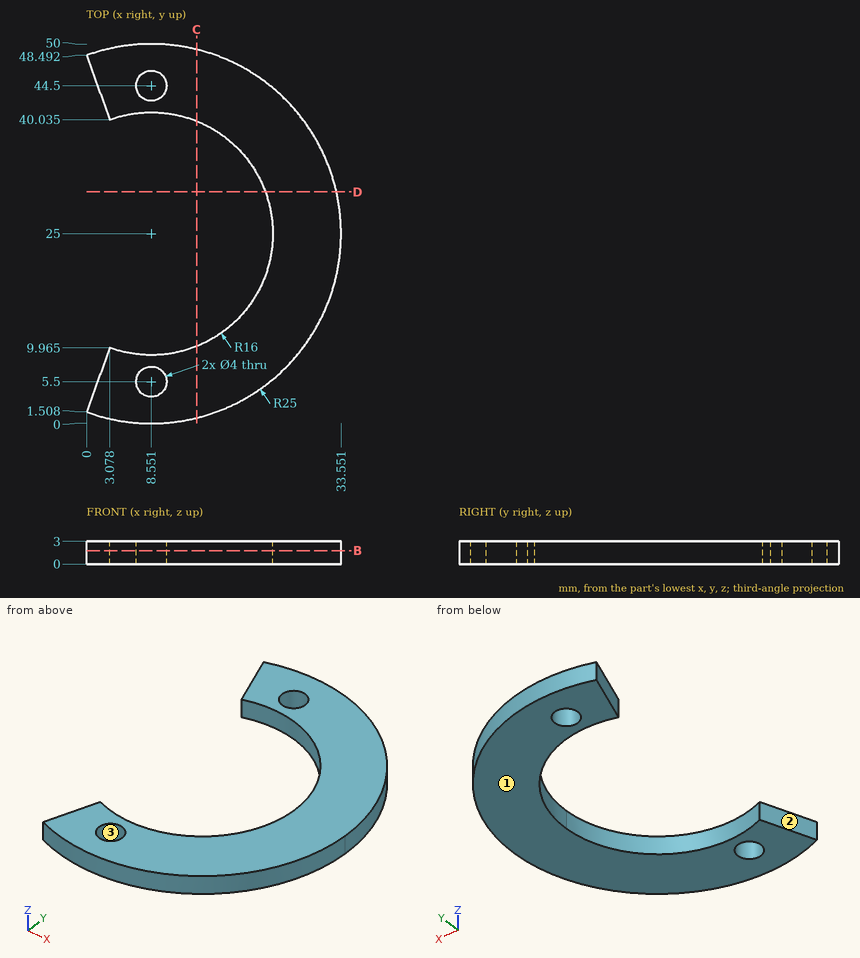
Here's the drawing with two shaded views (mm, measured from the low corner). I have some questions. Round coordinates to 2 decimals unless told otherwise and drop trailing zeros. Write each loop counter-clockwise with the first axis right and the second up, starting at its lowest first coordinate (ties: lowest second). Pieces come first, ordered by that corner, then holes. Notation, with made-up numbers: M 49,-28.75 L 75,-28.75 A16 ccw 75,-0.75 Z; hole C 9.5,-8.75 d2. An arc over 180 degrees is marked long. Write each question's results on one line, items separated by ' | '. Start each with the question number.
1. Thinking about a two-plate mould opening in X: for the marked faces 1, 2 and 3, which applies, +X half, -X half, draft (parallel to the pull), parting line (faces both ways), or undercut?
2. Imagine slicing it at C-C on x = 14.5. List the corners of the cut face in (y, z) for me.
3. I'm going to push flat-ended pins straight in: pin 1 Ø1 at (y, z) = (41.5, 2) entering from +X; pin 2 Ø3.5 at (x, y) = (8.55, 5.5) entering from +Z. Where does each tip first touch, or does it pass through?
4. Imagine slicing it at D-D on y = 30.5. List the corners of the cut face in (x, z) for me (1 decimal), and give its area (3 significant figures).
5. Imagine slicing it at B-B on z = 1.8. Count the separate pieces of the cut face and the enclosed holes in it, and give its area (3 significant figures).
6. I need wall thicknesses on L1, parallel to Y at x = 20.5, z = 0.7; L2, parallel to Y at x = 13, z = 1.6; L3, parallel to Y at x = 26, z = 1.95 (1 decimal). Which ranges of each line are inside material? Lowest first, please. Write a range as from..to.
Result sheet:
1) face 1: draft | face 2: -X half | face 3: undercut
2) outline: M 0.72,0 L 10.15,0 L 10.15,3 L 0.72,3 Z; M 39.85,0 L 49.28,0 L 49.28,3 L 39.85,3 Z
3) pin 1: stops at x = 27.76 | pin 2: passes through
4) outline: M 23.6,0 L 32.9,0 L 32.9,3 L 23.6,3 Z | area: 28.1 mm^2
5) separate pieces: 1 | enclosed holes: 2 | area: 683 mm^2
6) L1: y = 3.04..14.36, 35.64..46.96 | L2: y = 0.4..9.63, 40.37..49.6 | L3: y = 7.1..42.9
